The model under review builds one solid part; all positions refer to its coordinate system, in mm. Face numbers are marked on the shaded views. A direction names the side the tool comes from. Coordinates: 2 decimals unless noted, no trailing zeros. Order: outer loops, then holes, each group sorted by start corner. A loop starts at its lowest first (then second) coordinate and runs counter-clockwise, first axis right, second up. Notation, with made-up numbers: (28.25, 34) -> (35.25, 34) arc R20 ccw to (35.25, 72) -> close; hole circle Ø10 at (6.5, 80.25). An arc over 180 degrees is marked (long way). Use one line per item in the form item = value. Start each with the question number.
(1) Insertion check: pin 1 Ø4 at (x, z) = (-32, 41.5) entering from +Y; pin 2 Ø2.5 at (x, y) = (-5, 26.043) entering from +Z (3 decimals); pin 3 Ø4.5 at (x, y) = (-52.188, 26.043) entering from +Z. Each pin has a flat end and moves straight along its axis. Give the tip position at first contact, or say it passes through.
(2) Take a section at C-C (y = 29.75). State the section outline as (x, z) points.
(3) Take a section at A-A (x = -5). State the section outline as (y, z) points, then the cut area to 3 significant figures.
(4) Wall thickness on line 1 along X through (y, z) = (28.5, 36.5); line 2 along X through (y, z) = (26.75, 37.75); line 3 along X through (y, z) = (25, 43.25): over which ranges is each line inside the solid? List them lowest first.
(5) For the marked faces 4 and 5, list the 3-axis set-ups (+Z, -Z, +X, -X, +Y, -Y) from which the entire face can be reached by the end or side of a thin tool; tool diameter is ignored.
(6) Mouldability with a two-part tool opening along X and no side actions: class the marked faces 1, 2 and 3 as +X half, -X half, draft (parallel to the pull), parting line (faces both ways), or undercut.
(7) Take a section at D-D (x = -50). State the section outline as (y, z) points, then the cut area to 3 significant figures.
(8) Take a section at B-B (z = 39.5). State the section outline as (x, y) points, then the cut area to 3 significant figures.
Autodesk Inventor part; units mm, degrees
ref_plane "YZ Plane" through (0, 0, 0) normal (1, 0, 0) x (0, 1, 0)
ref_plane "XZ Plane" through (0, 0, 0) normal (0, 1, 0) x (-1, 0, 0)
ref_plane "XY Plane" through (0, 0, 0) normal (0, 0, 1) x (1, 0, 0)
ref_plane "Work Plane1" through (-28.594, 4.5215, 35.749) normal (0, 0, 1) x (1, 0, 0)
sketch "Sketch1" plane through (-28.594, 4.5215, 35.749) normal (0, 0, 1) x (1, 0, 0)
  circle A0 centre (23.594, 21.5215) radius 1.45
  circle A1 centre (-23.594, 21.5215) radius 1.45
  circle A2 centre (23.594, 21.5215) radius 1.45
  arc A3 (-26.094, 26.5215) -> (-28.594, 24.0215) centre (-26.094, 24.0215) ccw
  line L0 (26.094, 26.5215) -> (-26.094, 26.5215)
  arc A4 (28.594, 24.0215) -> (26.094, 26.5215) centre (26.094, 24.0215) ccw
  line L1 (28.594, 19.0215) -> (28.594, 24.0215)
  arc A5 (26.094, 16.5215) -> (28.594, 19.0215) centre (26.094, 19.0215) ccw
  line L2 (-26.094, 16.5215) -> (26.094, 16.5215)
  arc A6 (-28.594, 19.0215) -> (-26.094, 16.5215) centre (-26.094, 19.0215) ccw
  line L3 (-28.594, 24.0215) -> (-28.594, 19.0215)
  circle A7 centre (-23.594, 21.5215) radius 1.45
  point P0 (28.594, -4.5215)
extrude "Extrusion1" add sketch "Sketch1" along normal blind 7.842
sketch "Sketch2" plane through (-54.688, 31.043, 35.749) normal (0, 1, 0) x (1, 0, 0)
  line L0 (32.3438, -5.842) -> (19.8438, -5.842) construction
  line L1 (19.8438, -5.842) -> (19.8438, 0) construction
  line L2 (19.8438, 0) -> (32.3438, 0) construction
  line L3 (32.3438, 0) -> (32.3438, -5.842) construction
  line L4 (52.188, 0) -> (0, 0)
  line L5 (32.4438, 0) -> (32.4438, -6.017)
  line L6 (32.4438, -6.017) -> (19.7438, -6.017)
  line L7 (19.7438, -6.017) -> (19.7438, 0)
  point P0 (54.688, 35.749)
  dimension "d2" = 0.1
  dimension "d3" = 0.1
  dimension "d4" = 0.175
extrude "Extrusion2" cut sketch "Sketch2" against normal blind 12.908
ref_plane "Work Plane2" through (-52.188, -17, 42.6) normal (0, 0, -1) x (0, 1, 0)
sketch "Sketch3" plane through (-52.188, -17, 42.6) normal (0, 0, -1) x (0, 1, 0)
  line L0 (45.543, -5) -> (40.543, -5)
  arc A0 (38.043, -2.5) -> (40.543, -5) centre (40.543, -2.5) ccw
  line L1 (38.043, -2.5) -> (38.043, 49.688)
  arc A1 (40.543, 52.188) -> (38.043, 49.688) centre (40.543, 49.688) ccw
  line L2 (40.543, 52.188) -> (45.543, 52.188)
  arc A2 (48.043, 49.688) -> (45.543, 52.188) centre (45.543, 49.688) ccw
  line L3 (48.043, 49.688) -> (48.043, -2.5)
  arc A3 (45.543, -5) -> (48.043, -2.5) centre (45.543, -2.5) ccw
  circle A4 centre (43.043, 47.188) radius 1.45
  circle A5 centre (43.043, 0) radius 1.45
  circle A6 centre (0, 47.188) radius 3.065
  circle A7 centre (43.043, 47.188) radius 3.065
  circle A8 centre (43.043, 0) radius 3.065
  point P0 (17, 52.188)
extrude "Extrusion3" cut sketch "Sketch3" against normal blind 12.908 contours A4 | A5 | A7 | A8
properties part number "connectorHolder"
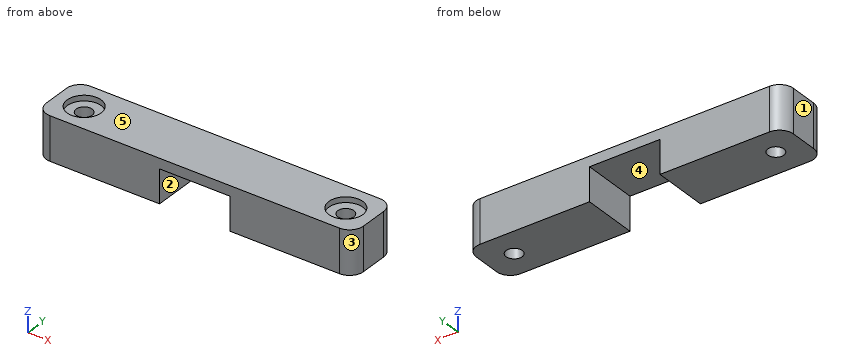
Findings:
q1.pin_1 = 31.04
q1.pin_2 = through
q1.pin_3 = 42.6
q2.outline = (-56.88, 35.75) -> (-34.94, 35.75) -> (-34.94, 41.77) -> (-22.24, 41.77) -> (-22.24, 35.75) -> (-0.31, 35.75) -> (-0.31, 43.59) -> (-56.88, 43.59) -> close
q3.outline = (21.04, 35.75) -> (24.59, 35.75) -> (24.59, 42.6) -> (22.98, 42.6) -> (22.98, 43.59) -> (21.04, 43.59) -> close; (27.49, 35.75) -> (31.04, 35.75) -> (31.04, 43.59) -> (29.11, 43.59) -> (29.11, 42.6) -> (27.49, 42.6) -> close
q3.area = 52.5 mm²
q4.line_1 = -57.19 to -34.94, -22.24 to 0
q4.line_2 = -57.19 to -53.45, -50.92 to -34.94, -22.24 to -6.27, -3.73 to 0
q4.line_3 = -57.19 to -55.07, -49.31 to -7.88, -2.12 to 0
q5.face_4 = -Z, +Y, -Y
q5.face_5 = +Z, +X, -X, +Y, -Y
q6.face_1 = -X half
q6.face_2 = undercut
q6.face_3 = +X half
q7.outline = (21.04, 35.75) -> (31.04, 35.75) -> (31.04, 43.59) -> (28.19, 43.59) -> (28.19, 42.6) -> (23.9, 42.6) -> (23.9, 43.59) -> (21.04, 43.59) -> close
q7.area = 74.2 mm²
q8.outline = (-57.19, 23.54) arc R2.5 ccw to (-54.69, 21.04) -> (-34.94, 21.04) -> (-34.94, 31.04) -> (-54.69, 31.04) arc R2.5 ccw to (-57.19, 28.54) -> close; (-22.24, 21.04) -> (-2.5, 21.04) arc R2.5 ccw to (0, 23.54) -> (0, 28.54) arc R2.5 ccw to (-2.5, 31.04) -> (-22.24, 31.04) -> close; hole circle Ø2.9 at (-52.19, 26.04); hole circle Ø2.9 at (-5, 26.04)
q8.area = 426 mm²
